The listing builds one solid part. Answer for the finished solid, in the listing's coordinates (mm). Give positions to 0.01 mm unless a question says otherwise; leave off trailing zeros. Loops run counter-clockwise (first coordinate to the right, second up) from the corner with the lowest first, then second, coordinate; pieces in that order, holes last.
Item 1: Each of these flat-tipped pins is pushed along its axis until it touches: pin 1 Ø3 at (y, z) = (0, 1) entering from -X; pin 2 Ø2 at (y, z) = (-1.5, 1.5) entering from -X; pin 3 Ø1 at (y, z) = (0, -1) entering from -X. Where does it stop, or does it pass through?
Item 2: Section A-A, the plane x = 4 is taken. Give the vertices of the cut face in (y, z).
Item 3: Consider line 1 along Z through (x, y) = (28.5, 1.6); line 2 along X through (y, z) = (0.9, -1.8); line 3 along Z through (x, y) = (43.5, 1.1) (3 decimals). Determine where each line is inside the solid, lowest interval first.
Item 4: Section B-B, the plane y = 1.5 is taken. Give the vertices of the cut face in (x, z), and give its area (3 significant figures).
Item 5: Section C-C, the plane z = -1.75 is taken. Give the vertices of the cut face in (x, y), and give its area (3 significant figures).
from build123d import *

# Parameters (mm, degrees)
F0_R     = 2.5
F1_DEPTH = 50
F2_R     = 2.5
F3_R     = 2.5


with BuildPart() as f1:
    # F0 (on Right) → F1 (new body)
    with BuildSketch(Plane.YZ):
        Circle(F0_R)
    extrude(amount=F1_DEPTH)

    # F2
    f2_edges = [f1.edges().sort_by_distance(p)[0] for p in [
        (50, -2.5, 0),
    ]]
    fillet(f2_edges, radius=F2_R)

    # F3
    f3_edges = [f1.edges().sort_by_distance(p)[0] for p in [
        (0, -2.5, 0),
    ]]
    fillet(f3_edges, radius=F3_R)


solid = f1.part
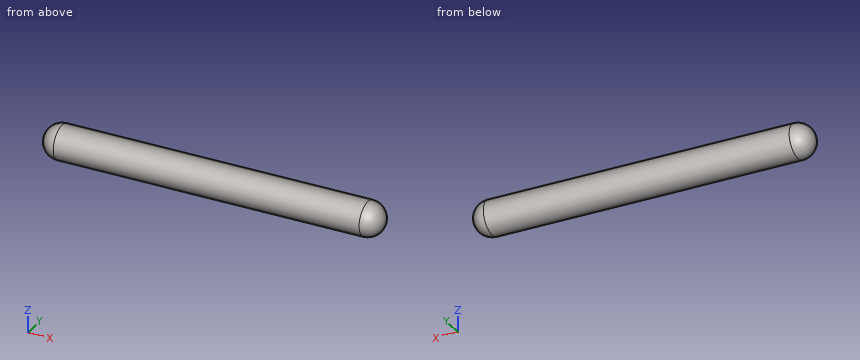
Worked answers:
1. pin 1: stops at x = 0
1. pin 2: stops at x = 0.27
1. pin 3: stops at x = 0.05
2. outline: circle Ø5 at (0, 0)
3. line 1: z = -1.92 to 1.92
3. line 2: x = 1.02 to 48.98
3. line 3: z = -2.245 to 2.245
4. outline: (2.5, -2) - (47.5, -2) arc R2 ccw to (47.5, 2) - (2.5, 2) arc R2 ccw to start
4. area: 193 mm2
5. outline: (2.5, -1.79) - (47.5, -1.79) arc R1.79 ccw to (47.5, 1.79) - (2.5, 1.79) arc R1.79 ccw to start
5. area: 171 mm2
